```python
from build123d import *

# Parameters (mm, degrees)
SKETCH1_R           = 32.5
SKETCH1_R_2         = 1
BOSS_EXTRUDE1_DEPTH = 3
BOSS_EXTRUDE2_START = 25
SKETCH3_R           = 32.5
SKETCH3_R_2         = 30.5
BOSS_EXTRUDE2_DEPTH = 25
BOSS_EXTRUDE3_DEPTH = 2


with BuildPart() as part:
    # Sketch1 → Boss-Extrude1 (new body)
    with BuildSketch(Plane(origin=(0, 0, 0), x_dir=(1, 0, 0), z_dir=(0, 1, 0))):
        with Locations(Location((0, 0, 0), (0, 0, 270))):
            Circle(SKETCH1_R)
        with Locations(Location((0, 0, 0), (0, 0, 270))):
            Circle(SKETCH1_R_2, mode=Mode.SUBTRACT)
    extrude(amount=BOSS_EXTRUDE1_DEPTH)

    # Sketch3 → Boss-Extrude2 (add)
    with BuildSketch(Plane.XZ.offset(BOSS_EXTRUDE2_START)):
        with Locations(Location((0, 0, 0), (0, 0, 270))):
            Circle(SKETCH3_R)
        with Locations(Location((0, 0, 0), (0, 0, 270))):
            Circle(SKETCH3_R_2, mode=Mode.SUBTRACT)
    extrude(amount=-BOSS_EXTRUDE2_DEPTH)

    # Sketch7 → Boss-Extrude3 (add)
    with BuildSketch(Plane.XZ.offset(25)):
        with BuildLine():
            ThreePointArc((4.775324886, 27.082213208), (0, -27.5), (-4.775324886, 27.082213208))
            Line((-4.775324886, 27.082213208), (-5.296269419, 30.036636467))
            ThreePointArc((-5.296269419, 30.036636467), (-19.605022095, -23.364355515), (30.5, 0))
            ThreePointArc((30.5, 0), (23.364355515, 19.605022095), (5.296269419, 30.036636467))
            Line((5.296269419, 30.036636467), (4.775324886, 27.082213208))
        make_face()
    extrude(amount=-BOSS_EXTRUDE3_DEPTH)


solid = part.part
```
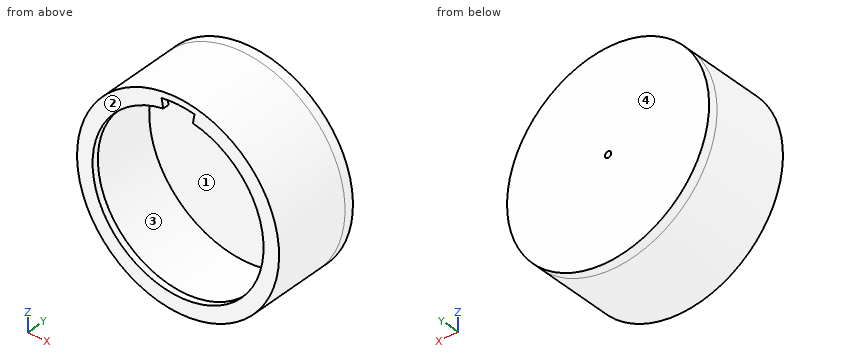
Verification items for the finished model (mm, model axes). Face numbers are marked on the shaded views. A direction names the side the tool comes from. Coordinates: 2 decimals unless noted, no trailing zeros. Order: outer loops, then holes, each group sorted by start corner. A loop starts at its lowest first (then second) coordinate and runs counter-clockwise, first axis right, second up. Notation, with made-up numbers: (-18.5, 54) -> (16.5, 54) arc R25 ccw to (16.5, 74) -> close; hole circle Ø9 at (-10.75, 87.5). An arc over 180 degrees is marked (long way). Answer as CSV lines item,"result". Start each with the question number.
1) Cross-section at B-B, the plane x = 0. Record the boundary of the cut face in (y, z), then the cut area to 3 significant figures.
2) Cross-section at C-C, the plane y = -14. Record the boundary of the cut face in (x, z), then the cut area to 3 significant figures.
3) Cross-section at D-D, the plane x = 21.5. Record the boundary of the cut face in (y, z).
4) Gauge pin test, flat ends, axial feed: pin 1 Ø4 at (x, y) = (-2.5, 0) entering from -Z; pin 2 Ø1 at (y, z) = (-7, -3.5) entering from -X; pin 3 Ø10 at (x, y) = (-9.5, -21.5) entering from -Z; pin 4 Ø8 at (x, y) = (-3, -5.5) entering from +Z. Record the tip position at first contact, or that the pin passes through.
5) Cross-section at A-A, the plane z = 0. Record the boundary of the cut face in (x, y).
6) Release check for a two-part mould opening along Z. For the marked faces 3 and 4 record: released by +Z, released by -Z, zero draft, split by the parting line, or undercut.
7) Set-up check for the marked faces 1 and 2: record each of +Z, -Z, +X, -X, +Y, -Y from which the full face is reachable in a straight line by a thin tool's end or side.
8) Material ranges on L1, parallel to X at y = -23.9, z = 0; L2, parallel to X at y = 2, z = 0; L3, parallel to Y at x = 7.5, z = 12.5, recorded low to high. Write a range as [from, to].
Conclusion:
1,outline,"(-25, -32.5) -> (3, -32.5) -> (3, -1) -> (0, -1) -> (0, -30.5) -> (-23, -30.5) -> (-23, -27.5) -> (-25, -27.5) -> close; (-25, 30.5) -> (0, 30.5) -> (0, 1) -> (3, 1) -> (3, 32.5) -> (-25, 32.5) -> close"
1,area,"295 mm²"
2,outline,"circle Ø65 at (0, 0); hole circle Ø61 at (0, 0)"
2,area,"396 mm²"
3,outline,"(-25, -24.37) -> (3, -24.37) -> (3, 24.37) -> (-25, 24.37) -> (-25, 17.15) -> (-23, 17.15) -> (-23, 21.63) -> (0, 21.63) -> (0, -21.63) -> (-23, -21.63) -> (-23, -17.15) -> (-25, -17.15) -> close"
4,pin 1,"stops at z = -32.5"
4,pin 2,"stops at x = -32.36"
4,pin 3,"stops at z = -32.19"
4,pin 4,"stops at z = 32.5"
5,outline,"(-32.5, -25) -> (-27.5, -25) -> (-27.5, -23) -> (-30.5, -23) -> (-30.5, 0) -> (-1, 0) -> (-1, 3) -> (-32.5, 3) -> close; (1, 0) -> (30.5, 0) -> (30.5, -23) -> (27.5, -23) -> (27.5, -25) -> (32.5, -25) -> (32.5, 3) -> (1, 3) -> close"
6,face 3,"undercut"
6,face 4,"zero draft"
7,face 1,"none"
7,face 2,"+Z, -Z, +X, -X, -Y"
8,L1,"x = [-32.5, -27.5], [27.5, 32.5]"
8,L2,"x = [-32.5, -1], [1, 32.5]"
8,L3,"y = [0, 3]"
